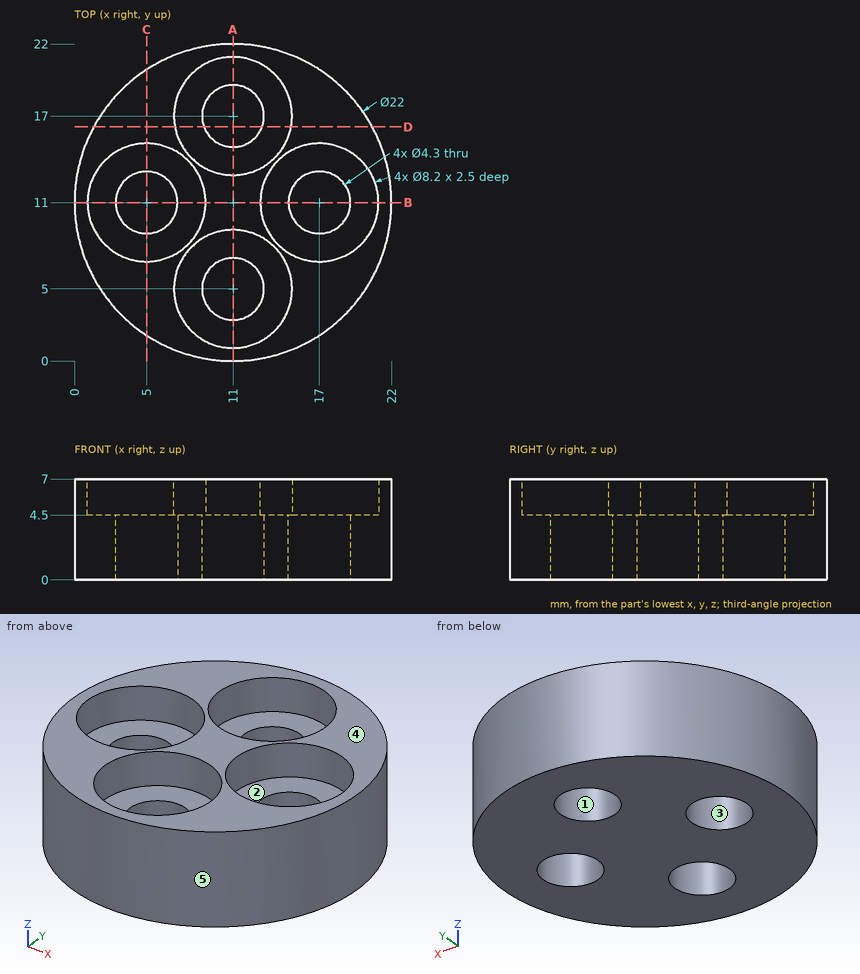
Job drawing, mm, ordinate dimensions from the low corner. One solid piece. A direction names the side the tool comes from. Give positions to 0.01 mm unless a question says otherwise; leave off trailing zeros. Write each loop counter-clockwise with the first axis right and the second up, starting at its lowest first coordinate (ties: lowest second). Pieces come first, ordered by that corner, then holes. Notation, with made-up numbers: (-31, 10.25) - (-5, 10.25) arc R21 ccw to (-5, 18.25) - close; hole circle Ø1 at (-9.75, 50.5). An arc over 180 degrees is marked (long way). Answer as CSV lines item,"result".
1. 3-axis set-ups, long thin cutter, end or side, ignore diameter. For the marked faces 1 and 2: which of +Z, -Z, +X, -X, +Y, -Y reach the whole face in a straight line?
Responses:
face 1,"+Z, -Z"
face 2,"+Z"
2. Band-saw the part on A-A (x = 11). Write the cut outline in (y, z).
Responses:
outline,"(0, 0) - (2.85, 0) - (2.85, 4.5) - (0.9, 4.5) - (0.9, 7) - (0, 7) - close; (7.15, 0) - (14.85, 0) - (14.85, 4.5) - (12.9, 4.5) - (12.9, 7) - (9.1, 7) - (9.1, 4.5) - (7.15, 4.5) - close; (19.15, 0) - (22, 0) - (22, 7) - (21.1, 7) - (21.1, 4.5) - (19.15, 4.5) - close"
3. Two-plate mould, pull along Y, no slides. Class the marked faces 3, 4 and 5: +Y half, -Y half, draft (parallel to the pull), parting line (faces both ways), or undercut.
Responses:
face 3,"undercut"
face 4,"draft"
face 5,"parting line"
4. Band-saw the part on C-C (x = 5). Write the cut outline in (y, z), and give its area (3 significant figures).
Responses:
outline,"(1.78, 0) - (8.85, 0) - (8.85, 4.5) - (6.9, 4.5) - (6.9, 7) - (1.78, 7) - close; (13.15, 0) - (20.22, 0) - (20.22, 7) - (15.1, 7) - (15.1, 4.5) - (13.15, 4.5) - close"
area,"89.2 mm2"
5. Band-saw the part on D-D (y = 16.25). Write the cut outline in (x, z), and give its area (3 significant figures).
Responses:
outline,"(1.33, 0) - (8.99, 0) - (8.99, 4.5) - (6.97, 4.5) - (6.97, 7) - (1.33, 7) - close; (13.01, 0) - (20.67, 0) - (20.67, 7) - (15.03, 7) - (15.03, 4.5) - (13.01, 4.5) - close"
area,"97.0 mm2"
6. Drill centre lines: L1, parallel to Y at x = 11, z = 6.4; L2, parallel to Y at x = 9.5, z = 3; L3, parallel to X at y = 12, z = 0.5. Where is each one in solid material? Low to high. Write a range as [from, to].
Responses:
L1,"y = [0, 0.9], [9.1, 12.9], [21.1, 22]"
L2,"y = [0.1, 3.46], [6.54, 15.46], [18.54, 21.9]"
L3,"x = [0.05, 3.1], [6.9, 15.1], [18.9, 21.95]"
7. Pin check, flat tips, straight feed: pin 1 (3.5 mm diameter, centred on x = 17, y = 11, fed in from +Z); pin 2 (4 mm diameter, centred on x = 11.5, y = 16, fed in from +Z); pin 3 (2 mm diameter, centred on x = 3.5, z = 1.5, fed in from +Y); pin 4 (3 mm diameter, centred on y = 4.5, z = 3.5, fed in from +X). Stop position of each tip, or through.
Responses:
pin 1,"passes through"
pin 2,"stops at z = 4.5"
pin 3,"stops at y = 19.87"
pin 4,"stops at x = 20.8"
